Model file for the job. Use its own axes, mm. A direction names the side the tool comes from. Coordinates: 2 decimals unless noted, no trailing zeros. Write each loop counter-clockwise with the first axis right and the second up, starting at its lowest first coordinate (ties: lowest second). Pieces come first, ordered by that corner, then holes.
Q1. Band-saw the part on A-A, the plane y = 38. Write the cut outline in (x, z), plus the area to 3 significant figures.
Q2. Band-saw the part on B-B, the plane z = -213.5. Write the cut outline in (x, y), plus the area to 3 significant figures.
Q3. Which spindle directions (+Z, -Z, +X, -X, +Y, -Y) get a long thin tool onto all of the face, cutting with end or side? Do faces 1 (the flat face through (-520, -63, -86.209)), 2 (the flat face through (-115.394, -63, -91)), 3 (the flat face through (432.273, 43, -355)). Say none if no direction does.
Q4. Pin check, flat tips, straight feed: P1, Ø1.6, axis at x = -605.5, y = -47, coming from the +Z side; P2, Ø2, axis at y = 27.5, z = -247, coming from the -X side; P3, Ø6, axis at x = -126.5, y = -48.5, coming from the -Z side. Stop position of each tip, or through.
Q5. Band-saw the part on D-D, the plane y = -91.5. Write the cut outline in (x, z).
Q6. Drill centre lines: probe 1 along X at (y, z) = (-52, -197); probe 2 along X at (y, z) = (13, -339.5); probe 3 along Y at (x, z) = (217.5, -379). Where is each one in solid material? Low to high.
Q7. Band-saw the part on C-C, the plane x = -462.5. Write the cut outline in (y, z).
Q8. Pull direction X, two halves, no side cores. Call faces 4 (the flat face through (-432.649, -63, -193)), 5 (the flat face through (604.993, -18, -313)), 6 (the flat face through (519.842, 79.688, -276.624)): released by +X, released by -X, zero draft, split by the parting line, or undercut.
from build123d import *

# Parameters (mm, degrees)
F0_W     = 172.344496
F0_H     = 210.44275
F1_DEPTH = 127
F4_DEPTH = 172.72
F5_DEPTH = 172.72


with BuildPart() as f1:
    # F0 (on Front) → F1 (new body)
    with BuildSketch(Plane.XZ):
        Polygon((0, 109.74871), (0, 0), (0, -296.65129), (115.393949, -296.65129), (115.393949, 109.74871), align=None)
        Polygon((0, -296.65129), (0, 0), (0, 109.74871), (-115.393949, 109.74871), (-115.393949, -296.65129), align=None)
        Polygon((115.393949, -296.65129), (0, -296.65129), (0, -461.782325), (604.993302, -461.782325), (604.993302, -296.65129), (432.648806, -296.65129), align=None)
        Polygon((0, -461.782325), (0, -296.65129), (-115.393949, -296.65129), (-432.648806, -296.65129), (-604.993302, -296.65129), (-606.454597, -296.65129), (-606.454597, -461.782325), align=None)
        with Locations((-518.821054, -191.429915)):
            Rectangle(F0_W, F0_H)
        with Locations((518.821054, -191.429915)):
            Rectangle(F0_W, F0_H)
    extrude(amount=F1_DEPTH)

    # F3 (on face) → F4 (join)
    with BuildSketch(Plane(origin=(-604.993302, 0, 0), x_dir=(0, -1, 0), z_dir=(-1, 0, 0))):
        Polygon((0, -462.243229), (0, -86.20854), (-158.201262, -462.243229), align=None)
    extrude(amount=-F4_DEPTH)

    # F2 (on face) → F5 (join)
    with BuildSketch(Plane.YZ.offset(604.993302)):
        Polygon((157.176092, -461.782325), (0, -86.20854), (0, -461.782325), align=None)
    extrude(amount=-F5_DEPTH)


solid = f1.part
Answer sheet:
1. outline: (-604.99, -462.24) - (-432.27, -462.24) - (-432.27, -176.53) - (-604.99, -176.53) - close; (432.27, -461.78) - (604.99, -461.78) - (604.99, -177.01) - (432.27, -177.01) - close
1. area: 98,500 mm2
2. outline: (-604.99, -127) - (-432.65, -127) - (-432.65, 0) - (-432.27, 0) - (-432.27, 53.55) - (-604.99, 53.55) - close; (-115.39, -127) - (115.39, -127) - (115.39, 0) - (-115.39, 0) - close; (432.27, 0) - (432.65, 0) - (432.65, -127) - (604.99, -127) - (604.99, 53.27) - (432.27, 53.27) - close
2. area: 91,500 mm2
3. face 1: +Z, -X, +Y, -Y
3. face 2: +Z, +Y, -Y
3. face 3: +Z, -Z, +Y
4. P1: stops at z = -86.21
4. P2: stops at x = -604.99
4. P3: stops at z = -461.78
5. outline: (-606.45, -461.78) - (604.99, -461.78) - (604.99, -86.21) - (432.65, -86.21) - (432.65, -296.65) - (115.39, -296.65) - (115.39, 109.75) - (-115.39, 109.75) - (-115.39, -296.65) - (-432.65, -296.65) - (-432.65, -86.21) - (-604.99, -86.21) - (-604.99, -296.65) - (-606.45, -296.65) - close
6. probe 1: x = -604.99 to -432.65, -115.39 to 115.39, 432.65 to 604.99
6. probe 2: x = -604.99 to -432.27, 432.27 to 604.99
6. probe 3: y = -127 to 0
7. outline: (-127, -461.78) - (0, -461.78) - (0, -462.24) - (158.2, -462.24) - (0, -86.21) - (-127, -86.21) - close
8. face 4: undercut
8. face 5: released by +X
8. face 6: zero draft
